The listing builds one solid part. Answer for the finished solid, in the listing's coordinates (mm). A direction names the side the tool comes from. Give positions to 0.01 mm unless a question says otherwise; leave off trailing zeros. Write each loop counter-clockwise with the first axis right and the second up, starting at its lowest first coordinate (ties: lowest second). Pieces come first, ordered by that corner, then holes.
```python
from build123d import *

# Parameters (mm, degrees)
ESQUISSE1_R                  = 3
BOSS_EXTRU_2_DEPTH           = 4
ESQUISSE2_R                  = 5
ESQUISSE2_R_2                = 2.25
BOSS_EXTRU_3_DEPTH           = 1
ESQUISSE3_R                  = 1
ENL_V_MAT_EXTRU_2_DEPTH      = 36.569219382
ENL_V_MAT_EXTRU_2_DEPTH_BACK = 3


with BuildPart() as part:
    # Esquisse1 → Boss.-Extru.2 (new body)
    with BuildSketch(Plane.XY):
        with BuildLine():
            Line((-30, 0), (30, 0))
            Line((30, 0), (30, 2))
            Line((30, 2), (24, 2))
            ThreePointArc((24, 2), (19, 3.339745962), (15.339745962, 7))
            Line((15.339745962, 7), (5.789084023, 23.542231724))
            ThreePointArc((5.789084023, 23.542231724), (4.528486677, 27.286561462), (4.81644602, 31.226890162))
            ThreePointArc((4.81644602, 31.226890162), (0, 37.569219382), (-4.81644602, 31.226890162))
            ThreePointArc((-4.81644602, 31.226890162), (-4.528486677, 27.286561462), (-5.789084023, 23.542231724))
            Line((-5.789084023, 23.542231724), (-15.339745962, 7))
            ThreePointArc((-15.339745962, 7), (-19, 3.339745962), (-24, 2))
            Line((-24, 2), (-30, 2))
            Line((-30, 2), (-30, 0))
        make_face()
        with Locations((0, 32.569219382)):
            Circle(ESQUISSE1_R, mode=Mode.SUBTRACT)
        with BuildLine():
            Line((-12.452994616, 2), (12.452994616, 2))
            ThreePointArc((12.452994616, 2), (14.185045424, 3), (14.185045424, 5))
            Line((14.185045424, 5), (1.732050808, 26.569219382))
            ThreePointArc((1.732050808, 26.569219382), (0, 27.569219382), (-1.732050808, 26.569219382))
            Line((-1.732050808, 26.569219382), (-14.185045424, 5))
            ThreePointArc((-14.185045424, 5), (-14.185045424, 3), (-12.452994616, 2))
        make_face(mode=Mode.SUBTRACT)
    extrude(amount=BOSS_EXTRU_2_DEPTH)

    # Esquisse2 → Boss.-Extru.3 (add)
    with BuildSketch(Plane.XY.offset(4)):
        with Locations((0, 32.569219382)):
            Circle(ESQUISSE2_R)
        with Locations((0, 32.569219382)):
            Circle(ESQUISSE2_R_2, mode=Mode.SUBTRACT)
    extrude(amount=-BOSS_EXTRU_3_DEPTH)

    # Esquisse3 → Enlèv. mat.-Extru.2 (cut, two sides)
    with BuildSketch(Plane(origin=(0, 2, 0), x_dir=(1, 0, 0), z_dir=(0, 1, 0))) as enl_v_mat_extru_2_sk:
        with Locations((27, -2)):
            Circle(ESQUISSE3_R)
        with Locations((-27, -2)):
            Circle(ESQUISSE3_R)
    extrude(amount=ENL_V_MAT_EXTRU_2_DEPTH, mode=Mode.SUBTRACT)
    extrude(enl_v_mat_extru_2_sk.sketch, amount=-ENL_V_MAT_EXTRU_2_DEPTH_BACK, mode=Mode.SUBTRACT)


solid = part.part
```
Item 1: A cutting plane is placed at B-B, the plane x = 0. Give the vertices of the cut face in (y, z), plus the area to 3 significant figures.
Conclusion:
outline: (0, 0) - (2, 0) - (2, 4) - (0, 4) - close; (27.57, 0) - (29.57, 0) - (29.57, 3) - (30.32, 3) - (30.32, 4) - (27.57, 4) - close; (34.82, 3) - (35.57, 3) - (35.57, 0) - (37.57, 0) - (37.57, 4) - (34.82, 4) - close
area: 25.5 mm2
Item 2: A cutting plane is placed at D-D, the plane y = 26. Give the vertices of the cut face in (x, z).
Conclusion:
outline: (-4.78, 0) - (-2.06, 0) - (-2.06, 4) - (-4.78, 4) - close; (2.06, 0) - (4.78, 0) - (4.78, 4) - (2.06, 4) - close
Item 3: Each of these flat-tipped pins is pushed along its axis until it touches: P1, Ø1.5, axis at y = 21, z = 3.5, coming from the -X side; P2, Ø3.5, axis at x = 0, y = 32.57, coming from the +Z side; P3, Ø2, axis at x = -28.5, z = 1.5, coming from the +Y side; P4, Ø3, axis at x = 1, y = 31.5, coming from the -Z side. Where does it stop, or does it pass through?
Conclusion:
P1: stops at x = -7.69
P2: passes through
P3: stops at y = 2
P4: stops at z = 3
Item 4: Which of the six approach directions +Z, -Z, +X, -X, +Y, -Y give full straight-line access (tool end or side, diameter ignored) to faces 1 (the face through (0, 35, 3)), 2 (the face through (26, 1, 2)), 3 (the face through (26, 2, 3)), 4 (the face through (-28, 2, 3)), 5 (the face through (14.17, 2.975, 1.972))?
Conclusion:
face 1: -Z
face 2: +Y, -Y
face 3: +Z, -Z, +X, +Y
face 4: +Z, -Z, -X, +Y
face 5: +Z, -Z
Item 5: A cutting plane is placed at A-A, the plane x = -27. Give the vertices of the cut face in (y, z), plus the area to 3 significant figures.
Conclusion:
outline: (0, 0) - (2, 0) - (2, 1) - (0, 1) - close; (0, 3) - (2, 3) - (2, 4) - (0, 4) - close
area: 4.00 mm2
Item 6: A cutting plane is placed at C-C, the plane z = 2. Give the vertices of the cut face in (x, y), plus the area to 3 significant figures.
Conclusion:
outline: (-30, 0) - (-28, 0) - (-28, 2) - (-30, 2) - close; (-26, 0) - (26, 0) - (26, 2) - (24, 2) arc R10 cw to (15.34, 7) - (5.79, 23.54) arc R10 cw to (4.82, 31.23) arc R5 ccw (long way) to (-4.82, 31.23) arc R10 cw to (-5.79, 23.54) - (-15.34, 7) arc R10 cw to (-24, 2) - (-26, 2) - close; (28, 0) - (30, 0) - (30, 2) - (28, 2) - close; hole (-14.19, 5) arc R2 ccw to (-12.45, 2) - (12.45, 2) arc R2 ccw to (14.19, 5) - (1.73, 26.57) arc R2 ccw to (-1.73, 26.57) - close; hole circle Ø6 at (0, 32.57)
area: 307 mm2
Item 7: Consider probe 1 along X at (y, z) = (1, 2); probe 2 along Y at (x, z) = (0, 1.95); probe 3 along Y at (x, z) = (0, 3.85). Determine where each line is inside the solid, lowest interval first.
Conclusion:
probe 1: x = -30 to -28, -26 to 26, 28 to 30
probe 2: y = 0 to 2, 27.57 to 29.57, 35.57 to 37.57
probe 3: y = 0 to 2, 27.57 to 30.32, 34.82 to 37.57
Item 8: Determine the mould class of faces 6 (the face through (-14.2, 3.03, 1.97)), 7 (the face through (-7.87, 15.94, 1.97)), 8 (the face through (-30, 1, 2)), 9 (the face through (-7, 19, 0)) for opening direction X: pulls with the +X half, pulls with the -X half, needs draft (parallel to the pull), parting line crosses it, or undercut.
Conclusion:
face 6: undercut
face 7: undercut
face 8: pulls with the -X half
face 9: needs draft
